from build123d import *

# Parameters (mm, degrees)
SKETCH1_W                       = 250
SKETCH1_H                       = 138
PLATE_DEPTH                     = 5
SKETCH2_W                       = 94.1
SKETCH2_H                       = 118
SKETCH2_W_2                     = 88.1
SKETCH2_H_2                     = 112
ARM_LOCATING_FENCE_DEPTH        = 4
SKETCH3_R                       = 1.7
ARM_M3_HOLES_DEPTH              = 7
SKETCH4_R                       = 1.7
DECK_M3_HOLES_DEPTH             = 7
SKETCH5_R                       = 3.25
DECK_COUNTERBORES_DEPTH         = 2.5
SKETCH6_W                       = 22.2
SKETCH6_H                       = 30.2
KILL_SWITCH_CUTOUT_DEPTH        = 7
SKETCH7_W                       = 12
SKETCH7_H                       = 30
SERVO_CABLE_SLOT_DEPTH          = 7
SKETCH8_R                       = 1.4
ESP32_STANDOFF_HOLES_M2P5_DEPTH = 7
SKETCH9_R                       = 3.5
MDD10A_BOSSES_DEPTH             = 6
SKETCH10_R                      = 1.3
MDD10A_PILOTS_M3_DEPTH          = 13
SKETCH11_W                      = 12
SKETCH11_H                      = 30
MOTOR_WIRE_SLOT_DEPTH           = 7
SKETCH12_W                      = 60
SKETCH12_H                      = 38
NAME_PLATE_RECESS_DEPTH         = 1.6


with BuildPart() as part:
    # Sketch1 → Plate (new body)
    with BuildSketch(Plane.XY.offset(98)):
        Rectangle(SKETCH1_W, SKETCH1_H)
    extrude(amount=PLATE_DEPTH)

    # Sketch2 → Arm_locating_fence (add)
    with BuildSketch(Plane.XY.offset(103)):
        with Locations((-65.85, 0)):
            Rectangle(SKETCH2_W, SKETCH2_H)
        with Locations((-65.85, 0)):
            Rectangle(SKETCH2_W_2, SKETCH2_H_2, mode=Mode.SUBTRACT)
    extrude(amount=ARM_LOCATING_FENCE_DEPTH)

    # Sketch3 → Arm_M3_holes (cut)
    with BuildSketch(Plane.XY.offset(97)):
        with Locations((-101.2, 31.7)):
            Circle(SKETCH3_R)
        with Locations((-101.2, -31.7)):
            Circle(SKETCH3_R)
        with Locations((-31.5, 27.8)):
            Circle(SKETCH3_R)
        with Locations((-31.5, -27.8)):
            Circle(SKETCH3_R)
    extrude(amount=ARM_M3_HOLES_DEPTH, mode=Mode.SUBTRACT)

    # Sketch4 → Deck_M3_holes (cut)
    with BuildSketch(Plane.XY.offset(97)):
        with Locations((-112, 63)):
            Circle(SKETCH4_R)
        with Locations((-112, -63)):
            Circle(SKETCH4_R)
        with Locations((112, 63)):
            Circle(SKETCH4_R)
        with Locations((112, -63)):
            Circle(SKETCH4_R)
    extrude(amount=DECK_M3_HOLES_DEPTH, mode=Mode.SUBTRACT)

    # Sketch5 → Deck_counterbores (cut)
    with BuildSketch(Plane.XY.offset(103)):
        with Locations((-112, 63)):
            Circle(SKETCH5_R)
        with Locations((-112, -63)):
            Circle(SKETCH5_R)
        with Locations((112, 63)):
            Circle(SKETCH5_R)
        with Locations((112, -63)):
            Circle(SKETCH5_R)
    extrude(amount=-DECK_COUNTERBORES_DEPTH, mode=Mode.SUBTRACT)

    # Sketch6 → Kill_switch_cutout (cut)
    with BuildSketch(Plane.XY.offset(97)):
        with Locations((102, -40)):
            Rectangle(SKETCH6_W, SKETCH6_H)
    extrude(amount=KILL_SWITCH_CUTOUT_DEPTH, mode=Mode.SUBTRACT)

    # Sketch7 → Servo_cable_slot (cut)
    with BuildSketch(Plane.XY.offset(97)):
        with Locations((-10.8, 0)):
            Rectangle(SKETCH7_W, SKETCH7_H)
    extrude(amount=SERVO_CABLE_SLOT_DEPTH, mode=Mode.SUBTRACT)

    # Sketch8 → ESP32_standoff_holes_M2p5 (cut)
    with BuildSketch(Plane.XY.offset(97)):
        with Locations((-6, -30)):
            Circle(SKETCH8_R)
        with Locations((-54, -30)):
            Circle(SKETCH8_R)
    extrude(amount=ESP32_STANDOFF_HOLES_M2P5_DEPTH, mode=Mode.SUBTRACT)

    # Sketch9 → MDD10A_bosses (add)
    with BuildSketch(Plane.XY.offset(103)):
        with Locations((13.13, 7.06)):
            Circle(SKETCH9_R)
        with Locations((13.13, 62.94)):
            Circle(SKETCH9_R)
        with Locations((91.87, 7.06)):
            Circle(SKETCH9_R)
        with Locations((91.87, 62.94)):
            Circle(SKETCH9_R)
    extrude(amount=MDD10A_BOSSES_DEPTH)

    # Sketch10 → MDD10A_pilots_M3 (cut)
    with BuildSketch(Plane.XY.offset(97)):
        with Locations((13.13, 7.06)):
            Circle(SKETCH10_R)
        with Locations((13.13, 62.94)):
            Circle(SKETCH10_R)
        with Locations((91.87, 7.06)):
            Circle(SKETCH10_R)
        with Locations((91.87, 62.94)):
            Circle(SKETCH10_R)
    extrude(amount=MDD10A_PILOTS_M3_DEPTH, mode=Mode.SUBTRACT)

    # Sketch11 → Motor_wire_slot (cut)
    with BuildSketch(Plane.XY.offset(97)):
        with Locations((104, 37)):
            Rectangle(SKETCH11_W, SKETCH11_H)
    extrude(amount=MOTOR_WIRE_SLOT_DEPTH, mode=Mode.SUBTRACT)

    # Sketch12 → Name_plate_recess (cut)
    with BuildSketch(Plane.XY.offset(102.4)):
        with Locations((45, -43)):
            Rectangle(SKETCH12_W, SKETCH12_H)
    extrude(amount=NAME_PLATE_RECESS_DEPTH, mode=Mode.SUBTRACT)


solid = part.part
Build history of the part. All positions in model axes, mm. A direction names the side the tool comes from. Round coordinates to 2 decimals unless told otherwise and drop trailing zeros. Write each loop counter-clockwise with the first axis right and the second up, starting at its lowest first coordinate (ties: lowest second). Pieces come first, ordered by that corner, then holes. Notation, with made-up numbers: M 51.5,-22.5 L 99.5,-22.5 A8 ccw 99.5,-7.5 Z; hole C 72.25,53.5 d11. An arc over 180 degrees is marked long. Answer as a JSON object with one key per item and string values. Group by question number.
(1) Cut at A-A (y = -7.5). Give the cut face in (x, z), and give its area (3 significant figures).
(2) Cut at B-B (x = -44). Give the cut face in (y, z).
(3) Drill centre lines: L1, parallel to Y at x = -112, z = 101.3; L2, parallel to X at y = -63, z = 99.3; L3, parallel to X at y = -51, z = 103.25. Where is each one in solid material? Low to high.
(4) Which spindle directions (+Z, -Z, +X, -X, +Y, -Y) get a long thin tool onto all of the face, cutting with end or side? Do faces 1 (the flat face through (113.1, -40, 100)), 2 (the flat face through (-2, -69, 100)), 3 (the flat face through (-110.6, -64.4, 100.5)). Say none if no direction does.
(5) Flat gauge pins, fed straight in: pin 1 (2 mm diameter, centred on x = 91.87, y = 62.94, fed in from +Z); pin 2 (7 mm diameter, centred on x = -110.5, y = 63, fed in from +Z); pin 3 (3 mm diameter, centred on x = -112.5, y = -62, fed in from +Z); pin 4 (3 mm diameter, centred on y = 8.5, z = 105.5, fed in from +X). Where does each tip first touch, or does it go through?
(6) Mould opens along X. For faces 4 (the flat face through (-11, 15, 100)), 5 (the flat face through (92, 61, 109)), 6 (the flat face through (104, 22, 100)) say: pulls with the +X half, pulls with the -X half, needs draft (parallel to the pull), parting line crosses it, or undercut.
Responses:
{
 "1": {"outline": "M -125,98 L -16.8,98 L -16.8,103 L -18.8,103 L -18.8,107 L -21.8,107 L -21.8,103 L -109.9,103 L -109.9,107 L -112.9,107 L -112.9,103 L -125,103 Z; M -4.8,98 L 125,98 L 125,103 L -4.8,103 Z", "area": "1,210 mm2"},
 "2": {"outline": "M -69,98 L 69,98 L 69,103 L 59,103 L 59,107 L 56,107 L 56,103 L -56,103 L -56,107 L -59,107 L -59,103 L -69,103 Z"},
 "3": {"L1": "y = -69 to -66.25, -59.75 to 59.75, 66.25 to 69", "L2": "x = -125 to -113.7, -110.3 to 110.3, 113.7 to 125", "L3": "x = -112.9 to -109.9, -21.8 to -18.8"},
 "4": {"face 1": "+Z, -Z", "face 2": "+Z, -Z, +X, -X, -Y", "face 3": "+Z"},
 "5": {"pin 1": "passes through", "pin 2": "stops at z = 103", "pin 3": "stops at z = 100.5", "pin 4": "stops at x = 95.37"},
 "6": {"face 4": "undercut", "face 5": "needs draft", "face 6": "undercut"}
}
